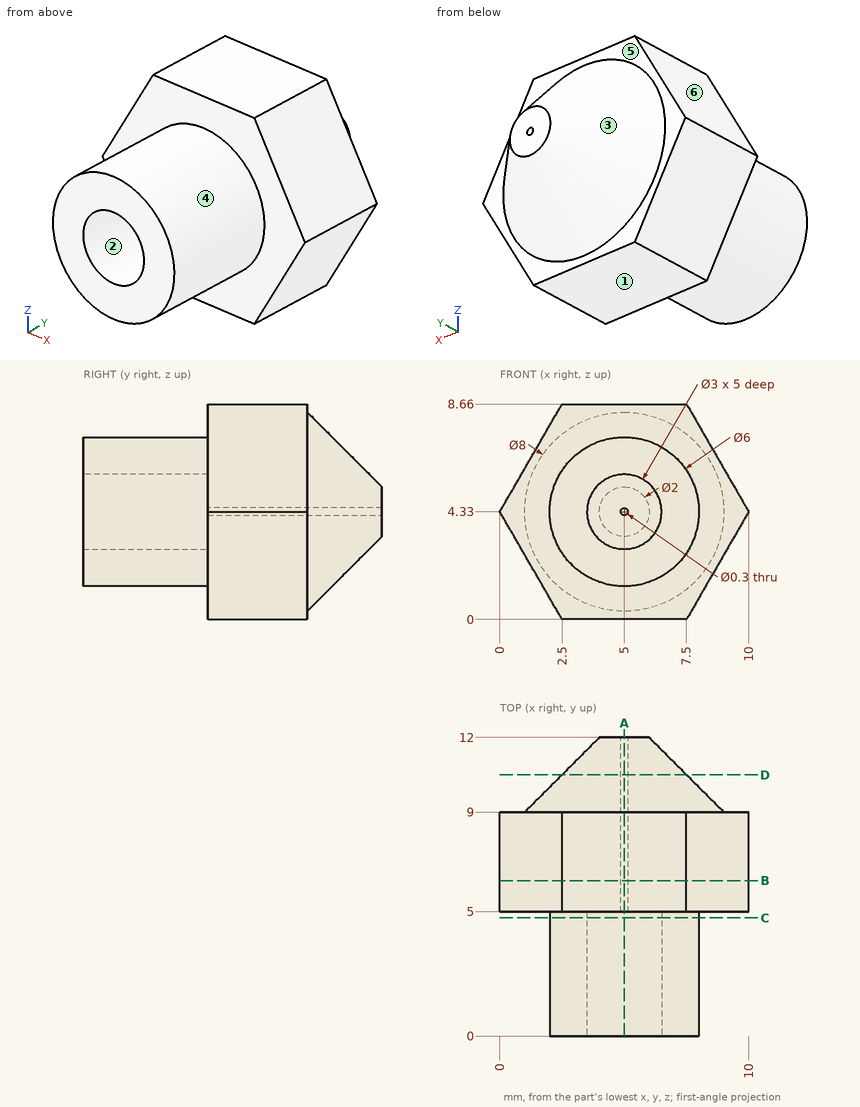
Design review of the part shown in the three views and the two pictorial views. Dimensions are in mm from the part's minimum x, y and z. A direction names the side the tool comes from. Round coordinates to 2 decimals unless told otherwise and drop trailing zeros. Order: outer loops, then holes, each group sorted by start corner. A loop starts at its lowest first (then second) coordinate and runs counter-clockwise, first axis right, second up.
Item 1: Draft analysis for pull direction X (two halves, no side actions). For the marked faces 1, 2 and 3, state which applies: released by +X, released by -X, zero draft, split by the parting line, or undercut.
Working result:
face 1: zero draft
face 2: undercut
face 3: split by the parting line
Item 2: Machinability: for the marked faces 4, 5 and 6, which of the approach directions +Z, -Z, +X, -X, +Y, -Y give a long, thin tool a straight path to every point of the face, cutting with its end or side? Answer none if there is none.
Working result:
face 4: -Y
face 5: +Y
face 6: +Z, -X, +Y, -Y
Item 3: Add section C-C, the plane y = 4.75. State the section outline as (x, z) points, and give its area (3 significant figures).
Working result:
outline: circle Ø6 at (5, 4.33); hole circle Ø3 at (5, 4.33)
area: 21.2 mm2
Item 4: To check wall thickness, follow probe 1 along X at (y, z) = (3, 4.25); probe 2 along Y at (x, z) = (7.5, 0.5); probe 3 along X at (y, z) = (0.5, 5.5). State the ranges of each line that lie inside material, in increasing order.
Working result:
probe 1: x = 2 to 3.5, 6.5 to 8
probe 2: y = 5 to 9
probe 3: x = 2.24 to 4.06, 5.94 to 7.76
Item 5: Add section A-A, the plane x = 5. State the section outline as (y, z) points.
Working result:
outline: (0, 1.33) - (5, 1.33) - (5, 0) - (9, 0) - (9, 0.33) - (12, 3.33) - (12, 4.18) - (5, 4.18) - (5, 2.83) - (0, 2.83) - close; (0, 5.83) - (5, 5.83) - (5, 4.48) - (12, 4.48) - (12, 5.33) - (9, 8.33) - (9, 8.66) - (5, 8.66) - (5, 7.33) - (0, 7.33) - close
Item 6: Add section B-B, the plane y = 6.25. State the section outline as (x, z) points.
Working result:
outline: (0, 4.33) - (2.5, 0) - (7.5, 0) - (10, 4.33) - (7.5, 8.66) - (2.5, 8.66) - close; hole circle Ø0.3 at (5, 4.33)
Item 7: Add section D-D, the plane y = 10.5. State the section outline as (x, z) points, and give its area (3 significant figures).
Working result:
outline: circle Ø5 at (5, 4.33); hole circle Ø0.3 at (5, 4.33)
area: 19.6 mm2
Item 8: For pin 1 (1.5 mm diameter, centred on x = 1.5, y = 6, fed in from +Z); pin 2 (0.9 mm diameter, centred on x = 5, z = 4, fed in from -Y); pin 3 (3 mm diameter, centred on x = 1, y = 3, fed in from +Z), all flat-tipped, find the tip position at first contact; note any pin that passes through.
Working result:
pin 1: stops at z = 8.23
pin 2: stops at y = 5
pin 3: stops at z = 5.99
